Can you work these out from the drawing? Everything is in mm from the part's minimum corner. A direction names the side the tool comes from. Coordinates: 2 decimals unless noted, no trailing zeros. Write each loop counter-clockwise with the first axis right and the second up, starting at its lowest first coordinate (ties: lowest second). Pieces come first, ordered by that corner, then holes. Notation, with made-up numbers: (11.25, -36.75) -> (18.25, -36.75) arc R13 ccw to (18.25, -27.75) -> close; hole circle Ø7 at (28.25, 57.5). An arc over 180 degrees is marked (long way). Use CSV: the item, a comma, the result in double quotes. Start each with the question number.
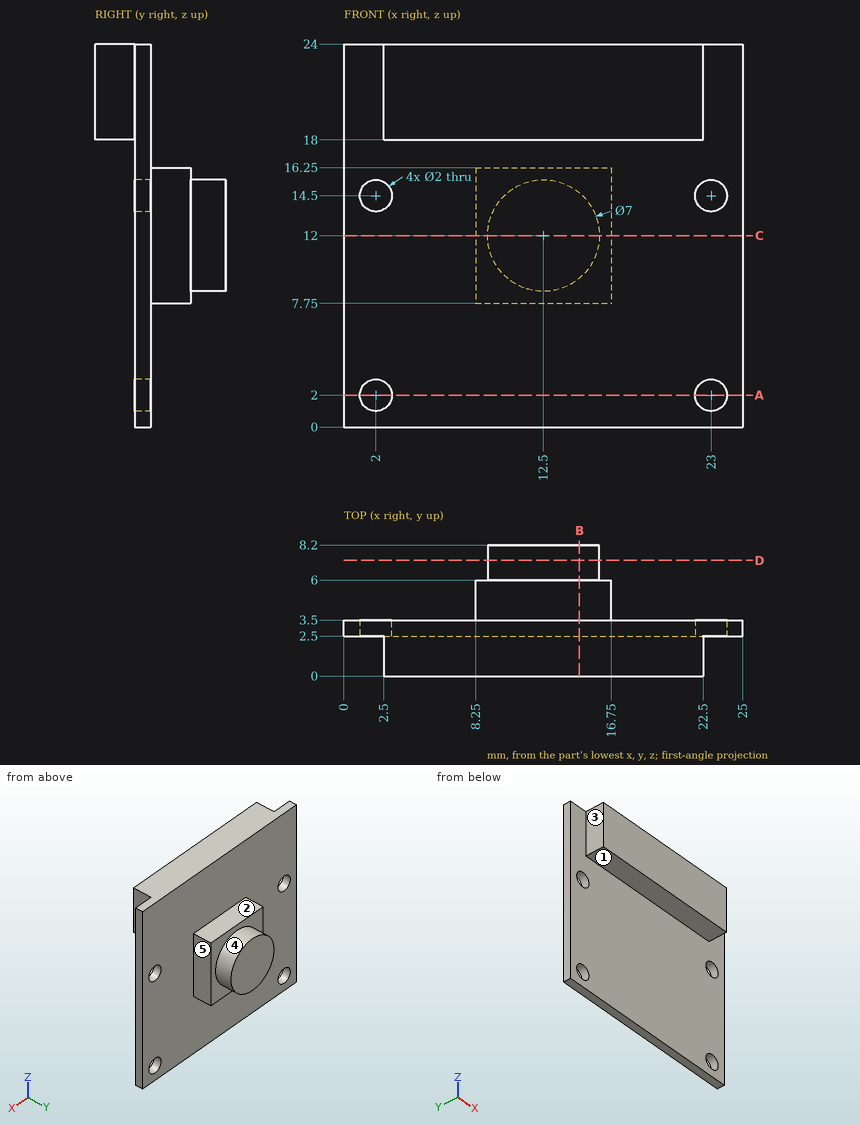
Item 1: I want a section at C-C on z = 12. Please give me the cut outline in (x, y), then the cut area to 4 significant figures.
Item 2: If I drill on line 1 along Z through (x, y) = (23, 2.9); line 2 along X through (y, z) = (2.8, 14.5); line 3 along Y through (x, z) = (18.75, 20.5), over which ranges is the centre line in solid material (lowest first)?
Item 3: I want a section at A-A on z = 2. Please give me the cut outline in (x, y), then the cut area to 3 significant figures.
Item 4: I want a section at D-D on y = 7.25. Please give me the cut outline in (x, z), then the cut area to 3 significant figures.
Item 5: I want a section at B-B on x = 14.75. Please give me the cut outline in (y, z), then the cut area to 3 significant figures.
Item 6: Which directions (+Z, -Z, +X, -X, +Y, -Y) give clear straight access to the entire face, cutting with the end or side of a thin tool? Please do the marked faces 1, 2, 3, 4 and 5.
Item 7: I'm going to push flat-ended pins straight in: pin 1 (2.5 mm diameter, centred on x = 2, z = 14.5, fed in from +Y); pin 2 (1.6 mm diameter, centred on x = 23, z = 14.5, fed in from +Y); pin 3 (2.5 mm diameter, centred on x = 23, z = 2, fed in from -Y); pin 4 (0.8 mm diameter, centred on x = 14.5, y = 5, fed in from +Z). Where does each tip first touch, or does it pass through?
Geometry says:
1,outline,"(0, 2.5) -> (25, 2.5) -> (25, 3.5) -> (16.75, 3.5) -> (16.75, 6) -> (16, 6) -> (16, 8.2) -> (9, 8.2) -> (9, 6) -> (8.25, 6) -> (8.25, 3.5) -> (0, 3.5) -> close"
1,area,"61.65 mm2"
2,line 1,"0 to 1, 3 to 13.5, 15.5 to 24"
2,line 2,"0 to 1, 3 to 22, 24 to 25"
2,line 3,"0 to 3.5"
3,outline,"(0, 2.5) -> (1, 2.5) -> (1, 3.5) -> (0, 3.5) -> close; (3, 2.5) -> (22, 2.5) -> (22, 3.5) -> (3, 3.5) -> close; (24, 2.5) -> (25, 2.5) -> (25, 3.5) -> (24, 3.5) -> close"
3,area,"21.0 mm2"
4,outline,"circle Ø7 at (12.5, 12)"
4,area,"38.5 mm2"
5,outline,"(0, 18) -> (2.5, 18) -> (2.5, 0) -> (3.5, 0) -> (3.5, 7.75) -> (6, 7.75) -> (6, 9.32) -> (8.2, 9.32) -> (8.2, 14.68) -> (6, 14.68) -> (6, 16.25) -> (3.5, 16.25) -> (3.5, 24) -> (0, 24) -> close"
5,area,"72.0 mm2"
6,face 1,"-Z, +X, -X, -Y"
6,face 2,"+Z, +X, -X, +Y"
6,face 3,"+Z, -Z, -X, -Y"
6,face 4,"+Y"
6,face 5,"+Z, -Z, +X, +Y"
7,pin 1,"y = 3.5"
7,pin 2,"through"
7,pin 3,"y = 2.5"
7,pin 4,"z = 16.25"
